For this review, take the finished solid that the model builds, in its own axes (mm). A direction names the side the tool comes from. Coordinates: 2 decimals unless noted, no trailing zeros. Write each loop counter-clockwise with the first axis right and the second up, starting at its lowest first coordinate (ties: lowest second). Pieces come first, ordered by that corner, then holes.
1) We need section C-C on y = 4.5. Write out the cut boundary in (x, z), then the cut area to 3 significant figures.
2) We need section B-B on z = 0. Write out the cut boundary in (x, y).
3) We need section A-A on x = 0. Write out the cut boundary in (y, z).
4) For faces 1 (the face through (0, 1, -4)), 2 (the face through (3, 6, 1)), list the 3-axis set-ups (+Z, -Z, +X, -X, +Y, -Y) from which the entire face can be reached by the end or side of a thin tool; tool diameter is ignored.
5) To check wall thickness, follow line 1 along Z through (x, y) = (0, 4); line 2 along Z through (x, y) = (-0.75, 5); line 3 along Z through (x, y) = (1, 0.5). State the ranges of each line that lie inside material, in increasing order.
6) Insertion check: P1, Ø3.5, axis at x = 0, y = 3, coming from the -Z side. The pin has a flat end and moves straight along its axis. Give the tip position at first contact, or say it passes through.
7) Mouldability with a two-part tool opening along X and no side actions: class faces 3 (the face through (2.53, 2.96, 1.61)), 4 (the face through (1.802, 2.958, 5.723)), 5 (the face through (-4, 5, 0)) as pulls with the +X half, pulls with the -X half, needs draft (parallel to the pull), parting line crosses it, or undercut.
8) We need section D-D on y = 0.75. Write out the cut boundary in (x, z), then the cut area to 3 significant figures.
from build123d import *

# Parameters (mm, degrees)
SKETCH_1_R          = 6
SKETCH_1_R_2        = 3
EXTRUDE_1_DEPTH     = 6
SKETCH_2_R          = 2
CUT_EXTRUDE_1_DEPTH = 10
SKETCH_3_R          = 2
CUT_EXTRUDE_2_DEPTH = 10


with BuildPart() as part:
    # 草图1 → 凸台-拉伸1 (new body)
    with BuildSketch(Plane(origin=(0, 0, 0), x_dir=(1, 0, 0), z_dir=(0, 1, 0))):
        with Locations(Location((0, 0, 0), (0, 0, 270))):
            Circle(SKETCH_1_R)
        with Locations(Location((0, 0, 0), (0, 0, 270))):
            Circle(SKETCH_1_R_2, mode=Mode.SUBTRACT)
    extrude(amount=EXTRUDE_1_DEPTH)

    # 草图2 → 切除-拉伸1 (cut)
    with BuildSketch(Plane.XY):
        with Locations(Location((0, 3, 0), (0, 0, 90))):
            Circle(SKETCH_2_R)
    extrude(amount=-CUT_EXTRUDE_1_DEPTH, mode=Mode.SUBTRACT)

    # 草图3 → 切除-拉伸2 (cut)
    with BuildSketch(Plane(origin=(0, 0, 0), x_dir=(0, 0, -1), z_dir=(1, 0, 0))):
        with Locations((0, 3)):
            Circle(SKETCH_3_R)
    extrude(amount=-CUT_EXTRUDE_2_DEPTH, mode=Mode.SUBTRACT)


solid = part.part
Result:
1. outline: (-5.85, -1.32) arc R6 ccw to (-1.32, -5.85) - (-1.32, -2.69) arc R3 cw to (-2.69, -1.32) - close; (-5.85, 1.32) - (-2.69, 1.32) arc R3 cw (long way) to (1.32, -2.69) - (1.32, -5.85) arc R6 ccw (long way) to start
1. area: 68.7 mm2
2. outline: (-6, 0) - (-3, 0) - (-3, 1) - (-6, 1) - close; (-6, 5) - (-3, 5) - (-3, 6) - (-6, 6) - close; (3, 0) - (6, 0) - (6, 6) - (3, 6) - close
3. outline: (0, -6) - (1, -6) - (1, -3) - (0, -3) - close; (0, 3) - (6, 3) - (6, 6) - (0, 6) - close; (5, -6) - (6, -6) - (6, -3) - (5, -3) - close
4. face 1: -Z
4. face 2: +Z, -Z, +X, -X, +Y
5. line 1: z = 3 to 6
5. line 2: z = -5.95 to -2.9, 2.9 to 5.95
5. line 3: z = -5.92 to -2.83, 2.83 to 5.92
6. P1: stops at z = 2.44
7. face 3: undercut
7. face 4: parting line crosses it
7. face 5: needs draft
8. outline: circle Ø12 at (0, 0); hole circle Ø6 at (0, 0)
8. area: 84.8 mm2
